Can you work these out from the model? Positions are in its coordinate system, mm. Face numbers are marked on the shaded views. Coordinates: 2 decimals unless noted, no trailing zeros. Loops run counter-clockwise (first coordinate to the right, second up) from the corner with the lowest first, then second, coordinate; pieces in that order, holes last. Notation, with made-up numbers: M 10.25,-13 L 61.25,-13 A25 ccw 61.25,9 Z; hole C 59.5,53.5 d11. An arc over 180 degrees is marked long. Answer as a JSON object with one key per item and string values. Group by question number.
Item 1: If I drill on line 1 (Y direction, x = 10, z = 7.5); line 2 (Y direction, x = -45, z = 1.75); line 3 (X direction, y = 73.5, z = 5.5), over which ranges is the centre line in solid material (lowest first)?
Item 2: Suppose I cut it at C-C (y = 0). Write out the boundary of the cut face in (x, z).
Item 3: I'm going to push flat-ended pins straight in: pin 1 Ø1.5 at (y, z) = (-51.5, 9) entering from -X; pin 2 Ø5 at (y, z) = (-54.5, 7) entering from -X; pin 3 Ø3 at (x, z) = (-69, 6) entering from -Y; pin 4 Ø6 at (x, y) = (-62.5, -71) entering from -Z. Where does each tip first touch, or does it pass through?
Item 4: We'd pull the mould along Y, two halves only. Please class the marked faces 1 and 2: +Y half, -Y half, draft (parallel to the pull), parting line (faces both ways), or undercut.
Item 5: Suppose I cut it at B-B (z = 4.25). Write out the boundary of the cut face in (x, y).
Item 6: Suppose I cut it at D-D (x = -58.5). Write out the boundary of the cut face in (y, z), then the cut area to 3 significant figures.
Item 7: Suppose I cut it at A-A (x = -2). Write out the boundary of the cut face in (y, z).
```python
from build123d import *

# Parameters (mm, degrees)
F1_DEPTH  = 10
F1_FACE_W = 2
F1_FACE_H = 10
F3_DEPTH  = 30
F4_DEPTH  = 30


with BuildPart() as f1:
    # F0 (on Top) → F1 (new body)
    with BuildSketch(Plane.XY):
        with BuildLine():
            Line((0, 88), (0, 90))
            ThreePointArc((0, 90), (-90, 0), (0, -90))
            Line((0, -90), (0, -88))
            ThreePointArc((0, -88), (-88, 0), (0, 88))
        make_face()
    extrude(amount=F1_DEPTH)

    # F1_face (on face) → F3 (join)
    with BuildSketch(Plane(origin=(0, -89, 5), x_dir=(0, 1, 0), z_dir=(1, 0, 0))):
        Rectangle(F1_FACE_W, F1_FACE_H)
    extrude(amount=F3_DEPTH)

    # F1_face (on face) → F4 (join)
    with BuildSketch(Plane(origin=(0, -89, 5), x_dir=(0, 1, 0), z_dir=(1, 0, 0))):
        with Locations((178, 0)):
            Rectangle(F1_FACE_W, F1_FACE_H)
    extrude(amount=F4_DEPTH)


solid = f1.part
```
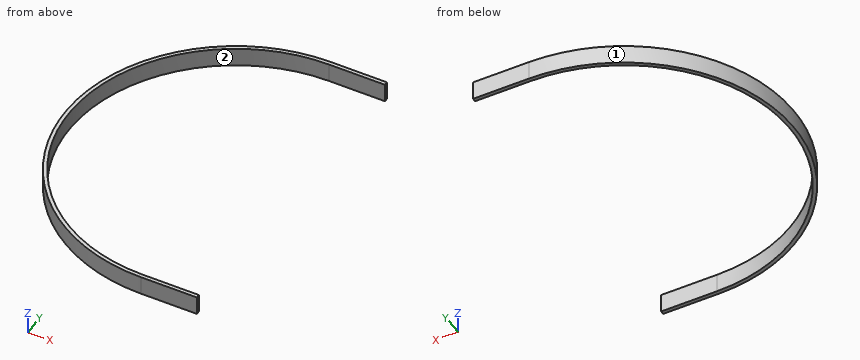
From the geometry:
{
 "1": {"line 1": "-90 to -88, 88 to 90", "line 2": "-77.94 to -75.62, 75.62 to 77.94", "line 3": "-51.94 to -48.39"},
 "2": {"outline": "M -90,0 L -88,0 L -88,10 L -90,10 Z"},
 "3": {"pin 1": "x = -74.33", "pin 2": "x = -73.46", "pin 3": "y = -59.53", "pin 4": "through"},
 "4": {"face 1": "parting line", "face 2": "undercut"},
 "5": {"outline": "M 0,-90 L 30,-90 L 30,-88 L 0,-88 A88 cw 0,88 L 30,88 L 30,90 L 0,90 A90 ccw Z"},
 "6": {"outline": "M -68.39,0 L -65.74,0 L -65.74,10 L -68.39,10 Z; M 65.74,0 L 68.39,0 L 68.39,10 L 65.74,10 Z", "area": "53.1 mm2"},
 "7": {"outline": "M -89.98,0 L -87.98,0 L -87.98,10 L -89.98,10 Z; M 87.98,0 L 89.98,0 L 89.98,10 L 87.98,10 Z"}
}
